```python
from build123d import *

# Parameters (mm, degrees)
TAGLIO_ESTRUSIONE1_DEPTH      = 12.258330249
TAGLIO_ESTRUSIONE1_DEPTH_BACK = 12.258330249
SCHIZZO2_W                    = 14.577161361
SCHIZZO2_H                    = 2.36968633
SCHIZZO2_H_2                  = 2.58511236
SCHIZZO3_R                    = 3
TAGLIO_ESTRUSIONE2_DEPTH      = 13.86468033
SMUSSO1_SIZE                  = 0.5


with BuildPart() as part:
    # Schizzo1 → Rivoluzione1 (revolve)
    with BuildSketch(Plane.XY):
        with BuildLine():
            Line((0, 6.5), (0, -6.5))
            ThreePointArc((0, -6.5), (-6.5, 0), (0, 6.5))
        make_face()
    revolve(axis=Axis((0, 8.58113686, 0), (0, -1, 0)))

    # Schizzo2 → Taglio-Estrusione1 (cut, two sides: drawn at the far end of the back side and taken through both)
    with BuildSketch(Plane.XY.offset(-TAGLIO_ESTRUSIONE1_DEPTH_BACK)):
        with Locations((0.181731429, 5.684843165)):
            Rectangle(SCHIZZO2_W, SCHIZZO2_H)
        with Locations((0.181731429, -5.79255618)):
            Rectangle(SCHIZZO2_W, SCHIZZO2_H_2)
    extrude(amount=TAGLIO_ESTRUSIONE1_DEPTH + TAGLIO_ESTRUSIONE1_DEPTH_BACK, mode=Mode.SUBTRACT)

    # Schizzo3 → Taglio-Estrusione2 (cut, through all)
    with BuildSketch(Plane(origin=(0, 4.5, 0), x_dir=(-1, 0, 0), z_dir=(0, 1, 0))):
        with Locations(Location((0, 0, 0), (0, 0, 90))):
            Circle(SCHIZZO3_R)
    extrude(amount=-TAGLIO_ESTRUSIONE2_DEPTH, mode=Mode.SUBTRACT)

    # Smusso1
    smusso1_edges = [part.edges().sort_by_distance(p)[0] for p in [
        (0, -4.5, -3),
        (0, 4.5, -3),
    ]]
    chamfer(smusso1_edges, length=SMUSSO1_SIZE)


solid = part.part
```
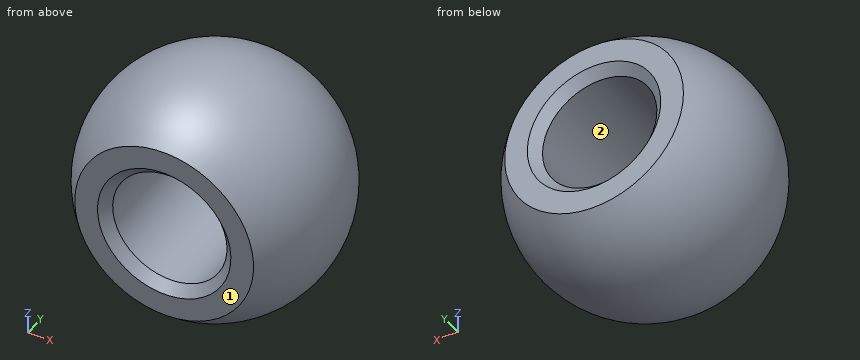
Input: part model. Units: mm. Frame: model coordinates. Face numbers are marked on the shaded views. Give positions to 0.01 mm unless a question says otherwise; leave off trailing zeros. Order: outer loops, then holes, each group sorted by start corner. A loop starts at its lowest first (then second) coordinate and runs counter-clockwise, first axis right, second up.
1. Pin query (flat end, axial travel): pin 1 (2 mm diameter, centred on x = -2.5, y = -1.5, fed in from -Z); pin 2 (5 mm diameter, centred on y = 2, z = -2, fed in from -X); pin 3 (1 mm diameter, centred on y = -2.5, z = -0.5, fed in from -X). Return the tip coordinate at first contact, or that it passes through.
Derived:
pin 1: stops at z = -6.21
pin 2: stops at x = -6.49
pin 3: stops at x = -6.17
2. Section C-C on y = 0. Return the cut outline in (x, z), and give its area (3 significant figures).
Derived:
outline: circle Ø13 at (0, 0); hole circle Ø6 at (0, 0)
area: 104 mm2
3. Section D-D on y = 2.5. Return the cut outline in (x, z), and give its area (3 significant figures).
Derived:
outline: circle Ø12 at (0, 0); hole circle Ø6 at (0, 0)
area: 84.8 mm2
4. Mould query, pull axis Z, two halves, no side actions, for the marked faces 1 and 2. Classes: released by +Z, released by -Z, zero draft, split by the parting line, or undercut.
Derived:
face 1: zero draft
face 2: undercut
5. Material intervals for L1, parallel to Z at x = 2, y = -2.5; L2, parallel to X at y = 1, z = 0; L3, parallel to X at y = 0.5, z = 0, sorted ascending.
Derived:
L1: z = -5.66 to -2.24, 2.24 to 5.66
L2: x = -6.42 to -3, 3 to 6.42
L3: x = -6.48 to -3, 3 to 6.48
6. Section B-B on x = 0. Return the cut outline in (y, z).
Derived:
outline: (-4.5, -4.69) arc R6.5 ccw to (4.5, -4.69) - (4.5, -3.5) - (4, -3) - (-4, -3) - (-4.5, -3.5) - close; (-4.5, 3.5) - (-4, 3) - (4, 3) - (4.5, 3.5) - (4.5, 4.69) arc R6.5 ccw to (-4.5, 4.69) - close
7. Section A-A on z = 0. Return the cut outline in (x, y), and give its area (3 significant figures).
Derived:
outline: (-4.69, -4.5) - (-3.5, -4.5) - (-3, -4) - (-3, 4) - (-3.5, 4.5) - (-4.69, 4.5) arc R6.5 ccw to start; (3, -4) - (3.5, -4.5) - (4.69, -4.5) arc R6.5 ccw to (4.69, 4.5) - (3.5, 4.5) - (3, 4) - close
area: 52.3 mm2
